```python
from build123d import *

# Parameters (mm, degrees)
ESBO_O1_W = 3
ESBO_O1_H = 23.6
ESBO_O2_W = 0.3
ESBO_O2_H = 0.5


with BuildPart() as part:
    # Esboço1 → Revolução1 (revolve)
    with BuildSketch(Plane.XY, mode=Mode.PRIVATE) as revolu_o1_sk:
        with Locations((-1.5, 0)):
            Rectangle(ESBO_O1_W, ESBO_O1_H)
    revolve(revolu_o1_sk.sketch.rotate(Axis((0, -11.8, 0), (0, 1, 0)), 180), axis=Axis((0, -11.8, 0), (0, 1, 0)))

    # Esboço2 → Corte-Revolução3 (revolve, cut)
    with BuildSketch(Plane.XY, mode=Mode.PRIVATE) as corte_revolu_o3_sk:
        with Locations((-2.85, -10.25)):
            Rectangle(ESBO_O2_W, ESBO_O2_H)
        with Locations((-2.85, 10.25)):
            Rectangle(ESBO_O2_W, ESBO_O2_H)
    revolve(corte_revolu_o3_sk.sketch.rotate(Axis((0, 0, 0), (0, 1, 0)), 270), axis=Axis((0, 0, 0), (0, 1, 0)), mode=Mode.SUBTRACT)


solid = part.part
```
Build history of the part. All positions in model axes, mm. A direction names the side the tool comes from. Round coordinates to 2 decimals unless told otherwise and drop trailing zeros. Write each loop counter-clockwise with the first axis right and the second up, starting at its lowest first coordinate (ties: lowest second). Pieces come first, ordered by that corner, then holes.
1) Pin check, flat tip, straight feed: pin 1 (3 mm diameter, centred on x = -0.5, y = -1.5, fed in from -Z). Stop position of the tip, or through.
2) Band-saw the part on A-A, the plane y = -8. List the corners of the cut face in (x, z), and give its area (3 significant figures).
3) Mould opens along Y. For faces 1 (the cylindrical face through (2.86, 11.16, -0.9)), 2 (the cylindrical face through (-0.811, -10.246, -2.575)), 3 (the flat face through (0, -11.8, 0)) say: +Y half, -Y half, draft (parallel to the pull), parting line (faces both ways), or undercut.
4) Band-saw the part on B-B, the plane z = -2.35. List the corners of the cut face in (x, y).
5) Band-saw the part on C-C, the plane x = 0.55. List the corners of the cut face in (y, z), and give its area (3 significant figures).
6) Drill centre lines: probe 1 along Y at (x, z) = (2.35, 1.65); probe 2 along X at (y, z) = (-8.5, -1.05); probe 3 along X at (y, z) = (8, -0.75). Where is each one in solid material? Low to high.
7) 3-axis set-ups, long thin cutter, end or side, ignore diameter. For faces 4 (the flat face through (0, 11.8, 0)), 5 (the cylindrical face through (-0.811, 10.254, -2.575)): which of +Z, -Z, +X, -X, +Y, -Y reach the whole face in a straight line?
Ans:
1. pin 1: stops at z = -3
2. outline: circle Ø6 at (0, 0)
2. area: 28.3 mm2
3. face 1: draft
3. face 2: undercut
3. face 3: -Y half
4. outline: (-1.86, -11.8) - (1.86, -11.8) - (1.86, -10.5) - (1.33, -10.5) - (1.33, -10) - (1.86, -10) - (1.86, 10) - (1.33, 10) - (1.33, 10.5) - (1.86, 10.5) - (1.86, 11.8) - (-1.86, 11.8) - (-1.86, 10.5) - (-1.33, 10.5) - (-1.33, 10) - (-1.86, 10) - (-1.86, -10) - (-1.33, -10) - (-1.33, -10.5) - (-1.86, -10.5) - close
5. outline: (-11.8, -2.95) - (-10.5, -2.95) - (-10.5, -2.64) - (-10, -2.64) - (-10, -2.95) - (10, -2.95) - (10, -2.64) - (10.5, -2.64) - (10.5, -2.95) - (11.8, -2.95) - (11.8, 2.95) - (10.5, 2.95) - (10.5, 2.64) - (10, 2.64) - (10, 2.95) - (-10, 2.95) - (-10, 2.64) - (-10.5, 2.64) - (-10.5, 2.95) - (-11.8, 2.95) - close
5. area: 139 mm2
6. probe 1: y = -11.8 to -10.5, -10 to 10, 10.5 to 11.8
6. probe 2: x = -2.81 to 2.81
6. probe 3: x = -2.9 to 2.9
7. face 4: +Z, -Z, +X, -X, +Y
7. face 5: none
